Design review of the part built by this model. Coordinates are the model's own, in mm. Face numbers are marked on the shaded views. A direction names the side the tool comes from. Coordinates: 2 decimals unless noted, no trailing zeros. Order: outer loops, then holes, each group sorted by start corner. A loop starts at its lowest first (then second) coordinate and runs counter-clockwise, first axis right, second up. Notation, with made-up numbers: M 52.25,43 L 58.25,43 A11 cw 58.25,62 Z; hole C 85,21.5 d6. An arc over 180 degrees is marked long. Answer as a JSON object with one key per item and string values.
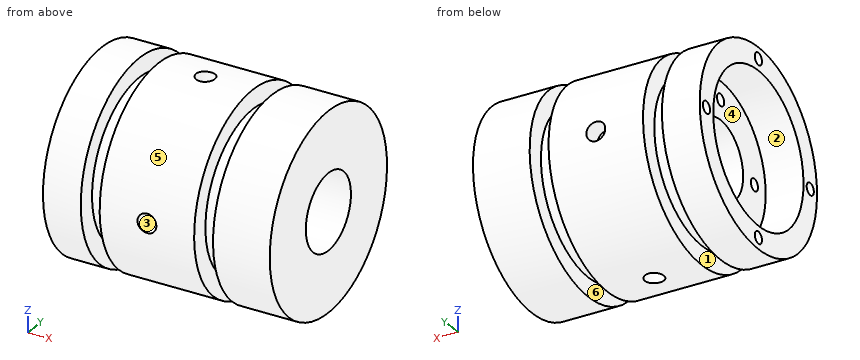
from build123d import *

# Parameters (mm, degrees)
SKETCH2_R                        = 20
CUT_EXTRUDE2_DEPTH               = 10
F_1_8_0_125_DIAMETER_HOLE1_D     = 3.175
F_1_8_0_125_DIAMETER_HOLE1_DEPTH = 7
F_1_8_0_125_DIAMETER_HOLE1_TIP   = 0.953866233
SKETCH6_R                        = 10
CUT_EXTRUDE3_DEPTH               = 50
F_1_2_0_5_DIAMETER_HOLE1_D       = 12.7
SKETCH10_R                       = 2.5
CUT_EXTRUDE8_DEPTH               = 5
SKETCH11_R                       = 2.5
CUT_EXTRUDE9_DEPTH               = 5
SKETCH12_R                       = 2.5
CUT_EXTRUDE10_DEPTH              = 5
SKETCH13_R                       = 2.5
CUT_EXTRUDE11_DEPTH              = 5
CUT_EXTRUDE12_START              = -5
SKETCH14_R                       = 2.5
CUT_EXTRUDE12_DEPTH              = 5
SKETCH15_R                       = 5
CUT_EXTRUDE13_DEPTH              = 103.225241501
SKETCH16_R                       = 45
CUT_EXTRUDE14_DEPTH              = 20
F_1_8_0_125_DIAMETER_HOLE2_D     = 3.175
F_1_8_0_125_DIAMETER_HOLE2_DEPTH = 7
F_1_8_0_125_DIAMETER_HOLE2_TIP   = 0.953866233


with BuildPart() as part:
    # Sketch1 → Revolve1 (revolve)
    with BuildSketch(Plane.XY, mode=Mode.PRIVATE) as revolve1_sk:
        Polygon((0, 0), (0, 26), (10, 26), (10, 21), (15, 21), (15, 26), (40, 26), (40, 21), (45, 21), (45, 26), (60, 26), (60, 45), (80, 45), (80, 0), align=None)
    revolve(revolve1_sk.sketch.rotate(Axis((0, 0, 0), (1, 0, 0)), 90), axis=Axis((0, 0, 0), (1, 0, 0)))

    # Sketch2 → Cut-Extrude2 (cut)
    with BuildSketch(Plane.ZY):
        Circle(SKETCH2_R)
    extrude(amount=-CUT_EXTRUDE2_DEPTH, mode=Mode.SUBTRACT)

    # 1/8 (0.125) Diameter Hole1
    with Locations(Plane.ZY.offset(-10)):
        with Locations((15.144669257, 0), (0.144669257, -15), (-14.855330743, 0), (0.144669257, 15)):
            Hole(F_1_8_0_125_DIAMETER_HOLE1_D / 2, depth=F_1_8_0_125_DIAMETER_HOLE1_DEPTH)
            with Locations((0, 0, -(F_1_8_0_125_DIAMETER_HOLE1_DEPTH + F_1_8_0_125_DIAMETER_HOLE1_TIP / 2))):  # 118° drill point
                Cone(0, F_1_8_0_125_DIAMETER_HOLE1_D / 2, F_1_8_0_125_DIAMETER_HOLE1_TIP, mode=Mode.SUBTRACT)

    # Sketch6 → Cut-Extrude3 (cut)
    with BuildSketch(Plane.ZY.offset(-10)):
        Circle(SKETCH6_R)
    extrude(amount=-CUT_EXTRUDE3_DEPTH, mode=Mode.SUBTRACT)

    # 1/2 (0.5) Diameter Hole1 (through all)
    with Locations(Plane(origin=(80, 0, 0), x_dir=(0, 0, -1), z_dir=(1, 0, 0))):
        with Locations((0, 0)):
            Hole(F_1_2_0_5_DIAMETER_HOLE1_D / 2)

    # Sketch10 → Cut-Extrude8 (cut)
    with BuildSketch(Plane(origin=(0, -26, 26), x_dir=(1, 0, 0), z_dir=(0, 0, 1))):
        with Locations((27.491787802, 26)):
            Circle(SKETCH10_R)
    extrude(amount=-CUT_EXTRUDE8_DEPTH, mode=Mode.SUBTRACT)

    # Sketch11 → Cut-Extrude9 (cut)
    with BuildSketch(Plane(origin=(0, 0, -26), x_dir=(-1, 0, 0), z_dir=(0, 0, -1))):
        with Locations((-27.5, 0)):
            Circle(SKETCH11_R)
    extrude(amount=-CUT_EXTRUDE9_DEPTH, mode=Mode.SUBTRACT)

    # Sketch12 → Cut-Extrude10 (cut)
    with BuildSketch(Plane(origin=(0, -26, 0), x_dir=(-1, 0, 0), z_dir=(0, -1, 0))):
        with Locations(Location((-27.5, 0, 0), (0, 0, 90))):
            Circle(SKETCH12_R)
    extrude(amount=-CUT_EXTRUDE10_DEPTH, mode=Mode.SUBTRACT)

    # Sketch13 → Cut-Extrude11 (cut)
    with BuildSketch(Plane(origin=(0, -21, 0), x_dir=(-1, 0, 0), z_dir=(0, -1, 0))):
        with Locations(Location((-27.5, 0, 0), (0, 0, 90))):
            Circle(SKETCH13_R)
    extrude(amount=-CUT_EXTRUDE11_DEPTH, mode=Mode.SUBTRACT)

    # Sketch14 → Cut-Extrude12 (cut)
    with BuildSketch(Plane(origin=(0, 26, 0), x_dir=(1, 0, 0), z_dir=(0, 1, 0)).offset(CUT_EXTRUDE12_START)):
        with Locations(Location((27.5, 0, 0), (0, 0, 90))):
            Circle(SKETCH14_R)
    extrude(amount=CUT_EXTRUDE12_DEPTH, mode=Mode.SUBTRACT)

    # Sketch15 → Cut-Extrude13 (cut, through all)
    with BuildSketch(Plane(origin=(80, 0, 0), x_dir=(0, 0, -1), z_dir=(1, 0, 0))):
        with Locations((0, -35)):
            Circle(SKETCH15_R)
        with Locations((-35, 0)):
            Circle(SKETCH15_R)
        with Locations((0, 35)):
            Circle(SKETCH15_R)
        with Locations((35, 0)):
            Circle(SKETCH15_R)
    extrude(amount=-CUT_EXTRUDE13_DEPTH, mode=Mode.SUBTRACT)

    # Sketch16 → Cut-Extrude14 (cut)
    with BuildSketch(Plane(origin=(80, 0, 0), x_dir=(0, 0, -1), z_dir=(1, 0, 0))):
        Circle(SKETCH16_R)
    extrude(amount=-CUT_EXTRUDE14_DEPTH, mode=Mode.SUBTRACT)

    # 1/8 (0.125) Diameter Hole2
    with Locations(Plane.ZY):
        with Locations((0, 23), (23, 0), (0, -23), (-23, 0)):
            Hole(F_1_8_0_125_DIAMETER_HOLE2_D / 2, depth=F_1_8_0_125_DIAMETER_HOLE2_DEPTH)
            with Locations((0, 0, -(F_1_8_0_125_DIAMETER_HOLE2_DEPTH + F_1_8_0_125_DIAMETER_HOLE2_TIP / 2))):  # 118° drill point
                Cone(0, F_1_8_0_125_DIAMETER_HOLE2_D / 2, F_1_8_0_125_DIAMETER_HOLE2_TIP, mode=Mode.SUBTRACT)


solid = part.part
1) Add section C-C (x = 27.5). State the section outline as (y, z) points.
Taken from the geometry:
{"outline": "M -25.88,-2.5 A26 ccw -2.5,-25.88 L -2.5,-21 L 2.5,-21 L 2.5,-25.88 A26 ccw 25.88,-2.5 L 21,-2.5 L 21,2.5 L 25.88,2.5 A26 ccw 2.5,25.88 L 2.5,21 L -2.5,21 L -2.5,25.88 A26 ccw -25.88,2.5 L -16,2.5 L -16,-2.5 Z; hole C 0,0 d20"}
2) Add section D-D (y = 17.5). State the section outline as (x, z) points, and give its area (3 significant figures).
Taken from the geometry:
{"outline": "M 0,-19.23 L 10,-19.23 L 10,-11.61 L 15,-11.61 L 15,-19.23 L 40,-19.23 L 40,-11.61 L 45,-11.61 L 45,-19.23 L 60,-19.23 L 60,19.23 L 45,19.23 L 45,11.61 L 40,11.61 L 40,19.23 L 15,19.23 L 15,11.61 L 10,11.61 L 10,19.23 L 0,19.23 L 0,9.68 L 10,9.68 L 10,-9.68 L 0,-9.68 Z", "area": "1,960 mm2"}
3) Mouldability with a two-part tool opening along Z and no side actions: class the marked faces 4, 5 and 6 as released by +Z, released by -Z, zero draft, split by the parting line, or undercut.
Taken from the geometry:
{"face 4": "undercut", "face 5": "split by the parting line", "face 6": "zero draft"}
4) Add section B-B (y = -6). State the section outline as (x, z) points.
Taken from the geometry:
{"outline": "M 0,-25.3 L 10,-25.3 L 10,-20.12 L 15,-20.12 L 15,-25.3 L 40,-25.3 L 40,-20.12 L 45,-20.12 L 45,-25.3 L 60,-25.3 L 60,-8 L 10,-8 L 10,-19.08 L 0,-19.08 Z; M 0,19.08 L 10,19.08 L 10,8 L 60,8 L 60,25.3 L 45,25.3 L 45,20.12 L 40,20.12 L 40,25.3 L 15,25.3 L 15,20.12 L 10,20.12 L 10,25.3 L 0,25.3 Z"}
5) Add section A-A (z = -4). State the section outline as (x, y) points, and give its area (3 significant figures).
Taken from the geometry:
{"outline": "M 0,-25.69 L 10,-25.69 L 10,-20.62 L 15,-20.62 L 15,-25.69 L 40,-25.69 L 40,-20.62 L 45,-20.62 L 45,-25.69 L 60,-25.69 L 60,-9.17 L 10,-9.17 L 10,-19.6 L 0,-19.6 Z; M 0,19.6 L 10,19.6 L 10,9.17 L 60,9.17 L 60,25.69 L 45,25.69 L 45,20.62 L 40,20.62 L 40,25.69 L 15,25.69 L 15,20.62 L 10,20.62 L 10,25.69 L 0,25.69 Z", "area": "1,670 mm2"}
6) Tool access review of the marked faces 1, 2 and 3: name each direction out of +Z, -Z, +X, -X, +Y, -Y from which nothing blocks a thin tool from reaching the whole face with its end or side.
Taken from the geometry:
{"face 1": "none", "face 2": "-X", "face 3": "-Y"}
7) To check wall thickness, follow L1, parallel to X at y = -18, z = -14; L2, parallel to Y at x = 3, z = 0; L3, parallel to Y at x = 7.5, z = 0. State the ranges of each line that lie inside material, in increasing order.
Taken from the geometry:
{"L1": "x = 0 to 10, 15 to 40, 45 to 60", "L2": "y = -26 to -24.59, -21.41 to -20, 20 to 21.41, 24.59 to 26", "L3": "y = -26 to -23.76, -22.24 to -20, 20 to 22.24, 23.76 to 26"}
8) Insertion check: pin 1 Ø1 at (x, y) = (22, -16) entering from +Z; pin 2 Ø6 at (x, y) = (48, 11) entering from -Z; pin 3 Ø2 at (x, z) = (50, -16.5) entering from -Y; pin 4 Ø5 at (y, z) = (-19.5, 13) entering from -X. Each pin has a flat end and moves straight along its axis. Give the tip position at first contact, or say it passes through.
Taken from the geometry:
{"pin 1": "stops at z = 20.87", "pin 2": "stops at z = -24.74", "pin 3": "stops at y = -20.87", "pin 4": "stops at x = 0"}
